Read the model definition and answer for the solid it produces. Units are mm, in the model's axes. A direction names the side the tool comes from. Round coordinates to 2 decimals unless told otherwise and drop trailing zeros. Write each loop counter-clockwise with the first axis right and the second up, starting at its lowest first coordinate (ties: lowest second). Pieces come first, ordered by that corner, then holes. Notation, with made-up numbers: (46, 35) - (100, 35) arc R33 cw to (100, 74) - close; hole circle Ø4 at (-38.5, 11.5). An arc over 180 degrees is marked (long way). One line per item, written item: value. Start each with the question number.
(1) A cutting plane is placed at C-C, the plane z = -112. Determine the outline of the cut face in (x, y).
(2) A cutting plane is placed at A-A, the plane x = 30.5. Determine the outline of the cut face in (y, z).
(3) Find the intervals of material crossed by L1, parallel to Z at x = 6.5, y = 51.5; L2, parallel to Z at x = -14, y = 10; L3, parallel to Y at x = 0, z = -126, in increasing order.
(4) The mould has two halves that part along Z. Classify faces 4 (the face through (-2, 41, 93.577)), 5 (the face through (-2, 82.55, 18)), 6 (the face through (-68.599, 41, 16)): +Z half, -Z half, draft (parallel to the pull), parting line (faces both ways), or undercut.
(5) A cutting plane is placed at B-B, the plane z = -42.5. Determine the outline of the cut face in (x, y).
(6) Flat-ended cylindrical pins translate along their axes: pin 1 Ø1.5 at (y, z) = (28.5, -72) entering from -X; pin 2 Ø5 at (x, y) = (44, 68) entering from -Z; pin 3 Ø25 at (x, y) = (5.5, 45.5) entering from -Z. Find the tip coordinate at first contact, or state that the pin passes through.
(7) For faces 1 (the face through (-4.13, 37.647, -106.408)), 2 (the face through (-1, 18, -168.043)), 3 (the face through (-2, 41, 91.037)), determine the directions among +Z, -Z, +X, -X, +Y, -Y from which every point of the face is accessible in a straight line to the end or side of a thin tool.
from build123d import *

# Parameters (mm, degrees)
F0_W        = 139.7
F0_H        = 152.4
F1_DEPTH    = 82.55
F2_R        = 19.05
F3_DEPTH    = 96.52
F4_R        = 3.81
F5_DEPTH    = 12.7
F6_T        = 2.54
F6_T4_ANGLE = 270.000000001
F6_T6_ANGLE = 90.000000001


# Not quite as in the source:
# - a shell that OpenCascade refuses in one call is made with other operations: the cavity is built on its own and cut out


with BuildPart() as f1:
    # F0 (on Front) → F1 (new body)
    with BuildSketch(Plane.XZ):
        with Locations((-1.2888036728, 17.3768577993)):
            Rectangle(F0_W, F0_H)
    extrude(amount=-F1_DEPTH)

    # F2 (on face) → F3 (join)
    with BuildSketch(Plane(origin=(0, 0, -58.8231422007), x_dir=(1, 0, 0), z_dir=(0, 0, -1))):
        with Locations((0, -19.05)):
            Circle(F2_R)
    extrude(amount=F3_DEPTH)

    # F4 (on face) → F5 (join)
    with BuildSketch(Plane(origin=(0, 0, -155.3431422007), x_dir=(1, 0, 0), z_dir=(0, 0, -1))):
        with Locations((0, -19.05)):
            Circle(F4_R)
    extrude(amount=F5_DEPTH)

    # F6: shell of thickness 2.54, made by hand


with BuildPart() as f6_core1:
    # F6_t2: copy of F1
    add(f1.part)

    # the walls: a layer under each face that stays
    f6_faces = [f6_core1.faces().sort_by_distance(p)[0] for p in [
        (-1.2888036728, 41.275, 93.5768577993),
        (68.5611963272, 41.275, 17.3768577993),
        (-71.1388036728, 41.275, 17.3768577993),
        (-1.2888036728, 0, 17.3768577993),
        (-1.2888036728, 82.55, 17.3768577993),
        (-1.2888036728, 41.275, -58.8231422007),
        (-19.05, 19.05, -107.0831422007),
        (-12.7, 31.75, -155.3431422007),
        (-3.81, 19.05, -161.6931422007),
    ]]
    thicken(f6_faces, amount=-F6_T, mode=Mode.SUBTRACT)

    # F6_s3 → F6_t4 (revolve, cut)
    with BuildSketch(Plane.YZ):
        Polygon((-0.0254, -58.8485422007), (0, -56.2831422007), (2.54, -56.2831422007), (2.54, -58.8231422007), align=None)
    revolve(axis=Axis((0, 19.05, -58.8231422007), (0, 0, -1)), revolution_arc=F6_T4_ANGLE, mode=Mode.SUBTRACT)

    # F6_s5 → F6_t6 (revolve, cut)
    with BuildSketch(Plane.XZ.offset(-19.05)):
        Polygon((19.0754, -58.8485422007), (19.05, -56.2831422007), (16.51, -56.2831422007), (16.51, -58.8231422007), align=None)
    revolve(axis=Axis((0, 19.05, -58.8231422007), (0, 0, -1)), revolution_arc=F6_T6_ANGLE, mode=Mode.SUBTRACT)

    # F6_s7 → F6_t8 (revolve, cut)
    with BuildSketch(Plane.XZ.offset(-19.05)):
        Polygon((3.8354, -155.3685422007), (3.81, -152.8031422007), (1.27, -152.8031422007), (1.27, -155.3431422007), align=None)
    revolve(axis=Axis((0, 19.05, -155.3431422007), (0, 0, -1)), mode=Mode.SUBTRACT)


with BuildPart() as f1_1:
    add(f1.part)

    # what is left inside the walls is the cavity
    f6_cavity = [f6_core1.part.solids().sort_by_distance(p)[0] for p in [
        (-1.288804, 79.9846, -7.176476),
    ]]
    add(f6_cavity, mode=Mode.SUBTRACT)


solid = f1_1.part
Here are the results:
1. outline: circle Ø38.1 at (0, 19.05); hole circle Ø33.02 at (0, 19.05)
2. outline: (0, -58.82) - (82.55, -58.82) - (82.55, 93.58) - (0, 93.58) - close; hole (2.54, -56.28) - (80.01, -56.28) - (80.01, 91.04) - (2.54, 91.04) - close
3. L1: -58.82 to -56.28, 91.04 to 93.58
3. L2: -155.34 to -56.28, 91.04 to 93.58
3. L3: 0 to 2.54, 35.56 to 38.1
4. face 4: +Z half
4. face 5: draft
4. face 6: undercut
5. outline: (-71.14, 0) - (68.56, 0) - (68.56, 82.55) - (-71.14, 82.55) - close; hole (-68.6, 2.54) - (66.02, 2.54) - (66.02, 80.01) - (-68.6, 80.01) - close
6. pin 1: x = -16.95
6. pin 2: z = -58.82
6. pin 3: z = -155.34
7. face 1: -Z
7. face 2: -Z, +X, -X, +Y, -Y
7. face 3: none
